Input: dimensioned drawing with shaded views. Units: mm. Origin: part minimum x, y, z. Round coordinates to 2 decimals unless told otherwise and drop trailing zeros. Loops run counter-clockwise (first coordinate to the right, second up) from the corner with the lowest first, then second, coordinate; pieces in that order, holes last. Notation, with made-up numbers: M -19,83 L 12,83 A29 cw 12,122 Z; hole C 25.25,40 d11. An arc over 180 degrees is marked long. Put each result on its own line as item: value. Start each with the question number.
1) Pin query (flat end, axial travel): pin 1 (2 mm diameter, centred on y = 27.5, z = 2, fed in from -X); pin 2 (2 mm diameter, centred on x = 29.5, z = 3.5, fed in from -Y); pin 3 (1.3 mm diameter, centred on y = 29.5, z = 2.5, fed in from +X). Return the tip coordinate at first contact, or that it passes through.
2) Section D-D on z = 2.15. Output: boundary loops of the cut face in (x, y).
3) Section A-A on x = 21.59. Output: boundary loops of the cut face in (y, z).
4) Section C-C on y = 6. Output: boundary loops of the cut face in (x, z), plus the area to 3 significant figures.
5) Section B-B on y = 38.5. Output: boundary loops of the cut face in (x, z).
6) Draft query along X for the marked faces 1 and 2. Return one class per face: +X half, -X half, draft (parallel to the pull), parting line (faces both ways), or undercut.
7) Line query: probe 1 along X at (y, z) = (22, 0.55); probe 2 along Z at (x, y) = (38.5, 31); probe 3 along Y at (x, z) = (21.59, 2.15). Output: solid intervals per line, ascending.
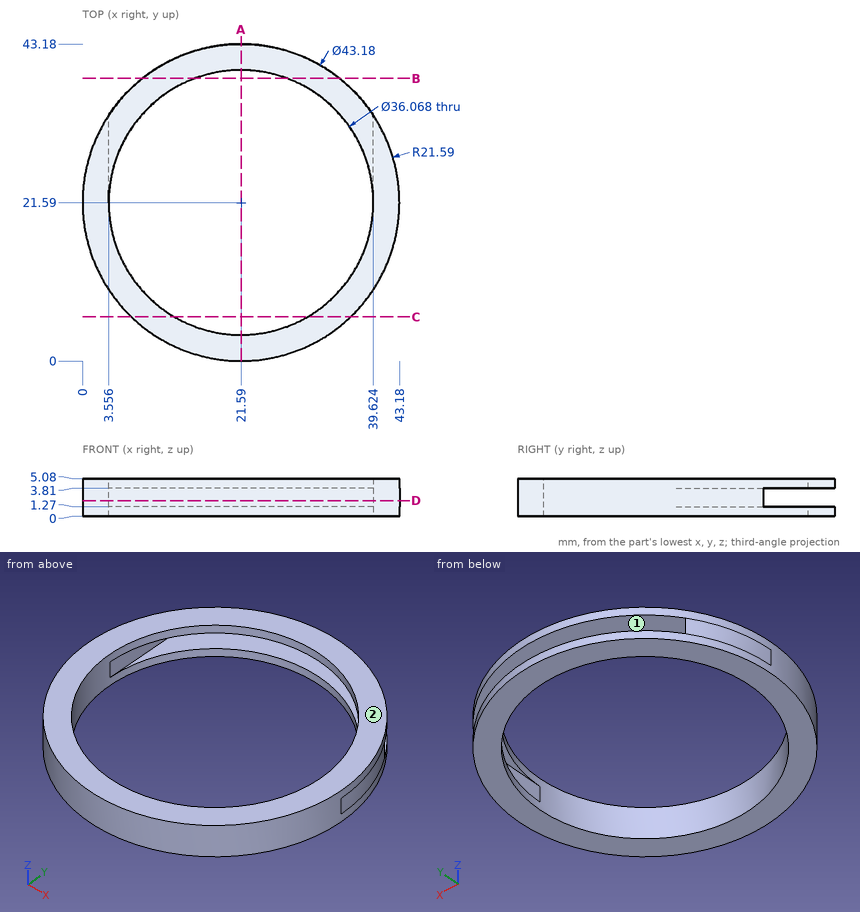
Geometry results:
1. pin 1: stops at x = 0.57
1. pin 2: stops at y = 1.14
1. pin 3: stops at x = 41.92
2. outline: M 3.56,21.59 L 3.56,33.46 A21.59 ccw long 39.62,33.46 L 39.62,21.59 A18.03 cw Z
3. outline: M 0,0 L 3.56,0 L 3.56,5.08 L 0,5.08 Z; M 39.62,0 L 43.18,0 L 43.18,1.27 L 39.62,1.27 Z; M 39.62,3.81 L 43.18,3.81 L 43.18,5.08 L 39.62,5.08 Z
4. outline: M 6.65,0 L 12.52,0 L 12.52,5.08 L 6.65,5.08 Z; M 30.66,0 L 36.53,0 L 36.53,5.08 L 30.66,5.08 Z
4. area: 59.6 mm²
5. outline: M 8.17,0 L 15.32,0 L 15.32,1.27 L 8.17,1.27 Z; M 8.17,3.81 L 15.32,3.81 L 15.32,5.08 L 8.17,5.08 Z; M 27.86,0 L 35.01,0 L 35.01,1.27 L 27.86,1.27 Z; M 27.86,3.81 L 35.01,3.81 L 35.01,5.08 L 27.86,5.08 Z
6. face 1: undercut
6. face 2: draft
7. probe 1: x = 0 to 3.56, 39.62 to 43.18
7. probe 2: z = 0 to 1.27, 3.81 to 5.08
7. probe 3: y = 0 to 3.56
